Here's how the part is built. I have some questions about the finished solid (model axes, mm). A direction names the side the tool comes from. Coordinates: 2 decimals unless noted, no trailing zeros. Write each loop counter-clockwise with the first axis right and the second up, starting at its lowest first coordinate (ties: lowest second). Pieces come first, ordered by that corner, then holes.
Item 1: If we section it at C-C (x = 58): Please give me the cut outline in (y, z).
Item 2: If we section it at B-B (z = -19.25): Please give me the cut outline in (x, y).
Item 3: I'm going to push flat-ended pins straight in: pin 1 Ø1 at (x, z) = (28, -19) entering from +Y; pin 2 Ø4 at (x, y) = (50.5, 10.5) entering from -Z; pin 3 Ø4.5 at (x, z) = (86.5, -1.5) entering from +Y. Where does each tip first touch, or does it pass through?
Item 4: For faces 1 (the face through (46, 4, -15)), 2 (the face through (86, 6.199, -2)), 3 (the face through (44, 2, -25)), which set-ups out of +Z, -Z, +X, -X, +Y, -Y let a thin tool reach every point of the face, with its end or its side?
Item 5: If we section it at A-A (x = 20): Please give me the cut outline in (y, z).
Item 6: If I drill on line 1 (Z direction, x = 28.5, y = 12.25); line 2 (Y direction, x = 7.5, z = -10); line 3 (Y direction, x = 71, z = -0.75), over which ranges is the centre line in solid material (lowest first)?
Item 7: If we section it at D-D (y = 14): Please give me the cut outline in (x, z), then the cut area to 3 significant figures.
from build123d import *

# Parameters (mm, degrees)
EXTRUDE_1_DEPTH     = 90
CUT_EXTRUDE_1_DEPTH = 26


with BuildPart() as part:
    # Эскиз1 → Вытянуть-Тонкостенный1 (new body)
    with BuildSketch(Plane(origin=(0, 0, 0), x_dir=(0, 0, -1), z_dir=(1, 0, 0))):
        Polygon((0, 25), (0, 0), (25, 0), (25, 4), (4, 4), (4, 25), align=None)
    extrude(amount=EXTRUDE_1_DEPTH)

    # Эскиз2 → Вырез-Вытянуть1 (cut, through all)
    with BuildSketch(Plane.XY):
        Polygon((0, 0), (0, 25), (25, 25), align=None)
        Polygon((90, 6.199303699), (81.394610848, 6.199303699), (62.593914547, 25), (90, 25), align=None)
    extrude(amount=-CUT_EXTRUDE_1_DEPTH, mode=Mode.SUBTRACT)


solid = part.part
Answer list:
1. outline: (0, -25) - (4, -25) - (4, -4) - (25, -4) - (25, 0) - (0, 0) - close
2. outline: (0, 0) - (90, 0) - (90, 4) - (4, 4) - close
3. pin 1: stops at y = 4
3. pin 2: stops at z = -4
3. pin 3: stops at y = 6.2
4. face 1: -Z, +X, -X, +Y
4. face 2: +Z, -Z, +X, +Y
4. face 3: -Z, +X, -X, +Y, -Y
5. outline: (0, -25) - (4, -25) - (4, -4) - (20, -4) - (20, 0) - (0, 0) - close
6. line 1: z = -4 to 0
6. line 2: y = 0 to 4
6. line 3: y = 0 to 16.59
7. outline: (14, -4) - (73.59, -4) - (73.59, 0) - (14, 0) - close
7. area: 238 mm2
